Geometry check sheet. Reference: the model listing, model coordinates, mm. Face numbers are marked on the shaded views. Coordinates: 2 decimals unless noted, no trailing zeros. Write each loop counter-clockwise with the first axis right and the second up, starting at its lowest first coordinate (ties: lowest second). Pieces come first, ordered by that corner, then holes. Notation, with made-up numbers: M 60.5,-20 L 78.5,-20 A11 ccw 78.5,-11 Z; hole C 15,49 d6. An arc over 180 degrees is marked long. Put each result on its own line as item: value. Start each with the question number.
1) Scan lines: line 1 along Z through (x, y) = (-450, 2037); line 2 along Y through (x, z) = (-609.5, -953). Record each from-to range of solid material in increasing order.
2) Mould release check, pull along Y, two halves, no side actions. Record for the marked faces 1, 2 and 3: released by +Y, released by -Y, zero draft, split by the parting line, or undercut.
3) Gauge pin test, flat ends, axial feed: pin 1 (3 mm diameter, centred on x = -348, z = -825, fed in from +Y); pin 2 (10 mm diameter, centred on x = -474.5, z = -151, fed in from -Y). Record the tip position at first contact, or that the pin passes through.
4) Cross-section at B-B on x = -613. Record the cut outline in (y, z).
5) Cross-section at D-D on y = 280. Record the cut outline in (x, z), plus the area to 3 significant figures.
6) Cross-section at A-A on y = 1743.5. Record the cut outline in (x, z).
7) Cross-section at C-C on z = -831. Record the cut outline in (x, y).
Autodesk Inventor part; units mm, degrees
ref_plane "YZ Plane" through (0, 0, 0) normal (1, 0, 0) x (0, 1, 0)
ref_plane "XZ Plane" through (0, 0, 0) normal (0, 1, 0) x (-1, 0, 0)
ref_plane "XY Plane" through (0, 0, 0) normal (0, 0, 1) x (1, 0, 0)
sketch "Sketch2" plane through (0, 0, 0) normal (0, 1, 0) x (-1, 0, 0)
  line L0 (0, 0) -> (900, 0)
  line L1 (900, 0) -> (900, -1000)
  line L2 (900, -1000) -> (0, -1000)
  line L3 (0, -1000) -> (0, 0)
  dimension "d0" = 900
  dimension "d1" = 1000
extrude "Extrusion1" add sketch "Sketch2" along normal blind 800
sketch "Sketch3" plane through (-900, 0, 0) normal (0, 0, 1) x (1, 0, 0)
  line L0 (900, 0) -> (0, 0)
  line L1 (0, 0) -> (100, 0)
  line L2 (900, 0) -> (900, 800)
  line L3 (900, 0) -> (800, 0)
  line L4 (800, 0) -> (100, 0)
  line L5 (100, 0) -> (100, 700)
  line L6 (100, 700) -> (800, 700)
  line L7 (800, 700) -> (800, 0)
  dimension "d4" = 100
  dimension "d5" = 100
  dimension "d6" = 700
extrude "Extrusion2" cut sketch "Sketch3" against normal through all
sketch "Sketch4" plane through (0, 0, 0) normal (1, 0, 0) x (0, 0, -1)
  line L0 (0, 0) -> (100, 0)
  line L1 (1000, 0) -> (0, 0)
  line L2 (1000, 0) -> (900, 0)
  line L3 (0, 700) -> (1000, 700)
  line L4 (900, 0) -> (100, 0)
  line L5 (100, 0) -> (100, 700)
  line L6 (100, 700) -> (900, 700)
  line L7 (900, 700) -> (900, 0)
  dimension "d9" = 100
  dimension "d10" = 100
extrude "Extrusion3" cut sketch "Sketch4" against normal through all
sketch "Sketch5" plane through (0, 0, 0) normal (0, -1, 0) x (1, 0, 0)
  line L0 (-900, -100) -> (-800, -100)
  line L1 (-800, -100) -> (-800, 0)
  line L2 (-900, 0) -> (-800, 0)
  line L3 (-900, -100) -> (-900, 0)
  line L4 (-800, -900) -> (-900, -900)
  line L5 (-900, -1000) -> (-900, -900)
  line L6 (-800, -1000) -> (-900, -1000)
  line L7 (-800, -1000) -> (-800, -900)
  line L8 (0, -900) -> (-100, -900)
  line L9 (-100, -900) -> (-100, -1000)
  line L10 (0, -1000) -> (-100, -1000)
  line L11 (0, -900) -> (0, -1000)
  line L12 (-100, -100) -> (0, -100)
  line L13 (0, 0) -> (0, -100)
  line L14 (-100, 0) -> (0, 0)
  line L15 (-100, 0) -> (-100, -100)
  line L16 (0, -100) -> (-100, -100)
  line L17 (0, -100) -> (100, -100)
  line L18 (100, -100) -> (100, 0)
  line L19 (100, 0) -> (0, 0)
  line L20 (0, 0) -> (0, -100)
  line L21 (0, -900) -> (100, -900)
  line L22 (100, -900) -> (100, -1000)
  line L23 (100, -1000) -> (0, -1000)
  line L24 (0, -1000) -> (0, -900)
  line L25 (-900, -1000) -> (-1000, -1000)
  line L26 (-1000, -1000) -> (-1000, -900)
  line L27 (-1000, -900) -> (-900, -900)
  line L28 (-900, -900) -> (-900, -1000)
  line L29 (-900, 0) -> (-1000, 0)
  line L30 (-1000, 0) -> (-1000, -100)
  line L31 (-1000, -100) -> (-900, -100)
  line L32 (-900, -100) -> (-900, 0)
  dimension "d13" = 100
  dimension "d14" = 100
extrude "Extrusion4" add sketch "Sketch5" against normal blind 2000 contours L31 L30 L29 L3 | L5 L25 L26 L27 | L21 L22 L23 L11 | L13 L19 L18 L17
sketch "Sketch6" plane through (0, 2000, 0) normal (0, 1, 0) x (1, 0, 0)
  line L0 (-1000, 1000) -> (-1000, 900)
  line L1 (100, 0) -> (100, 100)
  line L2 (-1000, 0) -> (-900, 0)
  line L3 (100, 1000) -> (100, 900)
  line L4 (100, 1000) -> (-100, 1000)
  line L5 (-1000, 0) -> (100, 0)
  line L6 (100, 0) -> (100, 1000)
  line L7 (100, 1000) -> (-1000, 1000)
  line L8 (-1000, 1000) -> (-1000, 0)
  line L9 (-1000, 0) -> (100, 1000) construction
  line L10 (100, 0) -> (-1000, 1000) construction
  line L11 (-1000, 1000) -> (-900, 1000)
  line L12 (-900, 1000) -> (-900, 0)
  line L13 (-900, 0) -> (-1000, 0)
  line L14 (-1000, 0) -> (-1000, 1000)
  line L15 (100, 0) -> (-1000, 0)
  line L16 (-1000, 0) -> (-1000, 100)
  line L17 (-1000, 100) -> (100, 100)
  line L18 (100, 100) -> (100, 0)
  line L19 (0, 1000) -> (100, 1000)
  line L20 (100, 1000) -> (100, 0)
  line L21 (100, 0) -> (0, 0)
  line L22 (0, 0) -> (0, 1000)
  line L23 (-1000, 900) -> (100, 900)
  line L24 (100, 900) -> (100, 1000)
  line L25 (100, 1000) -> (-1000, 1000)
  line L26 (-1000, 1000) -> (-1000, 900)
  line L27 (-1000, 900) -> (0, 0)
  line L28 (-900, 1000) -> (100, 100)
  line L29 (-1000, 100) -> (0, 1000)
  line L30 (-900, 0) -> (100, 900)
  point P0 (-450, 500)
  point P1 (-788.8889, 100)
  point P2 (-450, 405)
  point P3 (-111.1111, 100)
  point P4 (-100, 1000)
  point P5 (-111.1111, 900)
  point P6 (-450, 595)
  point P7 (-788.8889, 900)
  point P8 (0, 810)
  point P9 (0, 190)
  point P10 (-344.4444, 500)
  point P11 (-900, 190)
  point P12 (-900, 810)
  point P13 (-555.5556, 500)
extrude "Extrusion5" add sketch "Sketch6" along normal blind 50 contours L7 L12 L23 L0 | L27 L12 L29 L8 | L23 L12 L27 | L28 L23 L12 | L7 L4 L29 L23 L28 | L17 L12 L2 L8 | L29 L12 L17 | L23 L28 L29 L27 L12 | L17 L30 L12 | L12 L29 L27 L30 L17 | L29 L28 L30 L27 | L4 L3 L23 L22 | L22 L23 L29 | L23 L22 L30 L28 L29 | L30 L17 L27 L5 | L30 L28 L22 L17 L27 | L23 L30 L22 | L22 L17 L1 L5 | L27 L17 L22 | L6 L28 L22 L30 | L28 L17 L22
sketch "Sketch7" plane through (0, 2050, 0) normal (0, 1, 0) x (1, 0, 0)
  line L0 (-555.5556, 500) -> (-900, 190)
  line L1 (0, 190) -> (-344.4444, 500)
  line L2 (-555.5556, 500) -> (-344.4444, 500)
  line L3 (-111.1111, 900) -> (-450, 595)
  line L4 (-450, 405) -> (-111.1111, 100)
  line L5 (-450, 595) -> (-450, 405)
  circle A0 centre (-450, 500) radius 50
  circle A1 centre (-450, 500) radius 40
  point P0 (0, 0)
  dimension "d19" = 100
  dimension "d20" = 80
extrude "Extrusion6" cut sketch "Sketch7" against normal blind 200 contours A1 L5 L2 | L2 L5 A1 | L5 A1 L2 | L2 A1 L5
sketch "Sketch8" plane through (0, 2050, 0) normal (0, 1, 0) x (1, 0, 0)
  circle A0 centre (-450, 500) radius 40
  circle A1 centre (-450, 500) radius 60
  point P0 (0, 0)
  dimension "d23" = 120
extrude "Extrusion7" add sketch "Sketch8" along normal blind 100
properties part number "Soporte_Corte"
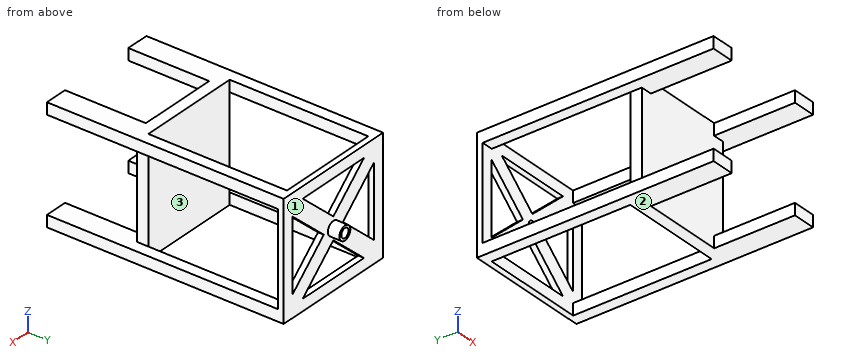
Answer key:
1. line 1: z = -1000 to -900, -595 to -540, -460 to -405, -100 to 0
1. line 2: y = 700 to 800, 2000 to 2050
2. face 1: released by +Y
2. face 2: zero draft
2. face 3: undercut
3. pin 1: stops at y = 800
3. pin 2: stops at y = 700
4. outline: M 700,-1000 L 800,-1000 L 800,0 L 700,0 Z; M 2000,-1000 L 2050,-1000 L 2050,-900 L 2000,-900 Z; M 2000,-741.7 L 2050,-741.7 L 2050,-551.7 L 2000,-551.7 Z; M 2000,-448.3 L 2050,-448.3 L 2050,-258.3 L 2000,-258.3 Z; M 2000,-100 L 2050,-100 L 2050,0 L 2000,0 Z
5. outline: M -1000,-1000 L -800,-1000 L -800,-900 L -1000,-900 Z; M -1000,-100 L -800,-100 L -800,0 L -1000,0 Z; M -100,-1000 L 100,-1000 L 100,-900 L -100,-900 Z; M -100,-100 L 100,-100 L 100,0 L -100,0 Z
5. area: 80,000 mm²
6. outline: M -1000,-1000 L -900,-1000 L -900,-900 L -1000,-900 Z; M -1000,-100 L -900,-100 L -900,0 L -1000,0 Z; M 0,-1000 L 100,-1000 L 100,-900 L 0,-900 Z; M 0,-100 L 100,-100 L 100,0 L 0,0 Z
7. outline: M -1000,2000 L -712.22,2000 L -712.22,2050 L -1000,2050 Z; M -900,700 L 0,700 L 0,800 L -900,800 Z; M -187.78,2000 L 100,2000 L 100,2050 L -187.78,2050 Z
